Autodesk Inventor part; units mm, degrees
ref_plane "YZ Plane" through (0, 0, 0) normal (1, 0, 0) x (0, 1, 0)
ref_plane "XZ Plane" through (0, 0, 0) normal (0, 1, 0) x (-1, 0, 0)
ref_plane "XY Plane" through (0, 0, 0) normal (0, 0, 1) x (1, 0, 0)
sketch "Sketch1" plane through (0, 0, 0) normal (0, 1, 0) x (-1, 0, 0)
  circle A0 centre (0, 0) radius 18.25
  dimension "d0" = 36.5
extrude "Extrusion1" add sketch "Sketch1" along normal blind 19.5
sketch "Sketch2" plane through (0, 19.5, 0) normal (0, 1, 0) x (1, 0, 0)
  circle A0 centre (0, 0) radius 8
  dimension "d3" = 16
extrude "Extrusion2" add sketch "Sketch2" along normal blind 2
sketch "Sketch3" plane through (0, 19.5, 0) normal (0, 1, 0) x (1, 0, 0)
  circle A0 centre (0, 21.95) radius 1.5
  circle A1 centre (0, -21.95) radius 1.5
  arc A2 (3.9863, 24.9682) -> (-3.9863, 24.9682) centre (0, 21.95) ccw
  circle A3 centre (0, 0) radius 8
  line L0 (-14.5499, -11.0165) -> (-3.9863, -24.9682)
  line L1 (-14.5499, 11.0165) -> (-3.9863, 24.9682)
  line L2 (14.5499, -11.0165) -> (3.9863, -24.9682)
  line L3 (14.5499, 11.0165) -> (3.9863, 24.9682)
  arc A4 (-14.5499, -11.0165) -> (14.5499, -11.0165) centre (0, 0) ccw
  arc A5 (3.0557, 17.9924) -> (-3.0557, 17.9924) centre (0, 0) ccw
  arc A6 (-3.9863, -24.9682) -> (3.9863, -24.9682) centre (0, -21.95) ccw
  arc A7 (3.0557, -17.9924) -> (-3.0557, -17.9924) centre (0, -21.95) ccw
  arc A8 (-14.5499, -11.0165) -> (14.5499, -11.0165) centre (0, 0) ccw
  arc A9 (14.5499, 11.0165) -> (-14.5499, 11.0165) centre (0, 0) ccw
extrude "Extrusion3" add sketch "Sketch3" against normal blind 2 contours L3 A9 A5 L1 A2 | A4 L2 A6 L0
sketch "Sketch4" plane through (0, 21.5, 0) normal (0, 1, 0) x (1, 0, 0)
  circle A0 centre (0, 0) radius 2.5
  dimension "d12" = 5
extrude "Extrusion4" add sketch "Sketch4" along normal blind 13
properties part number "14HM08"
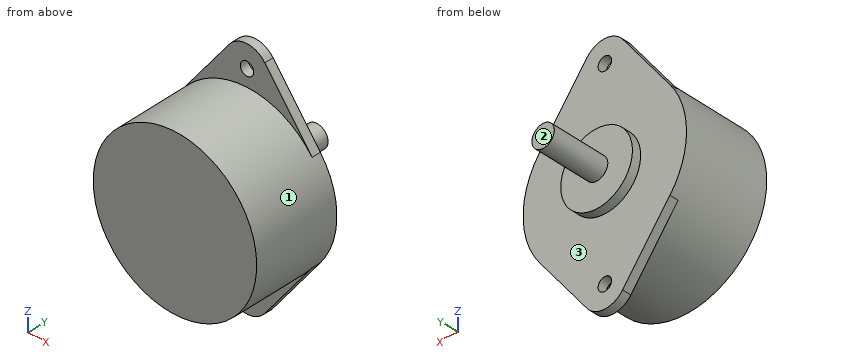
Design review of the part built by this model. Coordinates are the model's own, in mm. Face numbers are marked on the shaded views. A direction names the side the tool comes from. Give positions to 0.01 mm unless a question says otherwise; leave off trailing zeros. Order: outer loops, then holes, each group sorted by start corner. A loop starts at its lowest first (then second) coordinate and runs counter-clockwise, first axis right, second up. Notation, with made-up numbers: (60.5, -17) -> (73.5, -17) arc R30 cw to (73.5, 22) -> close; hole circle Ø9 at (13, 89.25). An arc over 180 degrees is marked (long way). Write each question's results on one line, items separated by ' | '. Start each with the question number.
Q1. Machinability: for the marked faces 1, 2 and 3, which of the approach directions +Z, -Z, +X, -X, +Y, -Y give a long, thin tool a straight path to every point of the face, cutting with its end or side? Answer none if there is none.
Q2. Add section D-D on y = 13.5. Give the boundary of the cut face in (x, z), and give its area (3 significant figures).
Q3. For pin 1 (3.5 mm diameter, centred on x = 0, z = -21.95, fed in from +Y); pin 2 (2 mm diameter, centred on x = 6.5, y = 20, fed in from -Z); pin 3 (4 mm diameter, centred on y = 9, z = -15, fed in from -X); pin 4 (12 mm diameter, centred on y = 22, z = 1.5, fed in from -X), all flat-tipped, find the tip position at first contact; note any pin that passes through.
Q4. Add section C-C on z = 0. Give the boundary of the cut face in (x, y), and give its area (3 significant figures).
Q5. Wall thickness on L1, parallel to Z at x = -11, y = 10; L2, parallel to Y at x = -5, z = 6; L3, parallel to X at y = 18.3, z = 21.95: over which ranges is each line inside the solid? List them lowest first. Write a range as from..to.
Q6. Add section B-B on z = -21.95. Give the boundary of the cut face in (x, y).
Q7. Add section A-A on x = 0. Give the boundary of the cut face in (y, z), and give its area (3 significant figures).
Found:
1) face 1: -Y | face 2: +Z, -Z, +X, -X, +Y | face 3: +Y
2) outline: circle Ø36.5 at (0, 0) | area: 1,050 mm2
3) pin 1: stops at y = 19.5 | pin 2: stops at z = -22.79 | pin 3: stops at x = -12.81 | pin 4: stops at x = -18.25
4) outline: (-18.25, 0) -> (18.25, 0) -> (18.25, 19.5) -> (8, 19.5) -> (8, 21.5) -> (2.5, 21.5) -> (2.5, 34.5) -> (-2.5, 34.5) -> (-2.5, 21.5) -> (-8, 21.5) -> (-8, 19.5) -> (-18.25, 19.5) -> close | area: 809 mm2
5) L1: z = -14.56..14.56 | L2: y = 0..21.5 | L3: x = -6.27..-1.5, 1.5..6.27
6) outline: (-6.27, 17.5) -> (-1.5, 17.5) -> (-1.5, 19.5) -> (-6.27, 19.5) -> close; (1.5, 17.5) -> (6.27, 17.5) -> (6.27, 19.5) -> (1.5, 19.5) -> close
7) outline: (0, -18.25) -> (17.5, -18.25) -> (17.5, -20.45) -> (19.5, -20.45) -> (19.5, -8) -> (21.5, -8) -> (21.5, -2.5) -> (34.5, -2.5) -> (34.5, 2.5) -> (21.5, 2.5) -> (21.5, 8) -> (19.5, 8) -> (19.5, 20.45) -> (17.5, 20.45) -> (17.5, 18.25) -> (0, 18.25) -> close; (17.5, -26.95) -> (19.5, -26.95) -> (19.5, -23.45) -> (17.5, -23.45) -> close; (17.5, 23.45) -> (19.5, 23.45) -> (19.5, 26.95) -> (17.5, 26.95) -> close | area: 832 mm2
